```python
from build123d import *

# Parameters (mm, degrees)
F0_W     = 25.4
F0_H     = 30.48
F1_DEPTH = 317.5
F0_W_2   = 20.8801385015
F0_H_2   = 34.5365251615
F2_DEPTH = 254
F3_R     = 76.2


with BuildPart() as f1:
    # F0 (on Front) → F1 (new body)
    with BuildSketch(Plane.XZ):
        Polygon((0, 121.8727435376), (-95.25, 62.9464942231), (95.25, 62.9464942231), align=None)
        Polygon((95.25, 62.9464942231), (-95.25, 62.9464942231), (-95.25, -62.9464942231), (-20.8801385015, -62.9464942231), (-20.8801385015, -28.4099690616), (0, -28.4099690616), (0, -62.9464942231), (95.25, -62.9464942231), align=None)
        with Locations((-49.3217527476, -33.6759798229)):
            Rectangle(F0_W, F0_H, mode=Mode.SUBTRACT)
        with Locations((52.5188967586, -33.6759798229)):
            Rectangle(F0_W, F0_H, mode=Mode.SUBTRACT)
        with Locations((-49.3217527476, 34.4667454919)):
            Rectangle(F0_W, F0_H, mode=Mode.SUBTRACT)
        with Locations((52.5188967586, 34.0303108096)):
            Rectangle(F0_W, F0_H, mode=Mode.SUBTRACT)
    extrude(amount=F1_DEPTH)

    # F0 (on Front) → F2 (join)
    with BuildSketch(Plane.XZ):
        with Locations((52.5188967586, 34.0303108096)):
            Rectangle(F0_W, F0_H)
        with Locations((-49.3217527476, 34.4667454919)):
            Rectangle(F0_W, F0_H)
        with Locations((52.5188967586, -33.6759798229)):
            Rectangle(F0_W, F0_H)
        with Locations((-49.3217527476, -33.6759798229)):
            Rectangle(F0_W, F0_H)
        with Locations((-10.4400692508, -45.6782316424)):
            Rectangle(F0_W_2, F0_H_2)
    extrude(amount=F2_DEPTH)

    # F3
    f3_edges = [f1.edges().sort_by_distance(p)[0] for p in [
        (0, -158.75, 121.872744),
    ]]
    fillet(f3_edges, radius=F3_R)


solid = f1.part
```
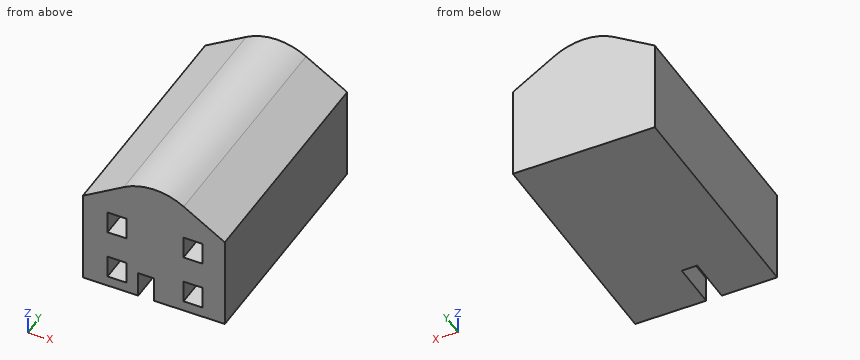
Part model, mm, in its own coordinate system. Give positions to 0.01 mm unless a question says otherwise; leave off trailing zeros. Order: outer loops, then holes, each group sorted by start corner. A loop starts at its lowest first (then second) coordinate and runs counter-clockwise, first axis right, second up. Notation, with made-up numbers: M 22.5,-16 L 39.5,-16 A38 cw 39.5,22 Z; hole C 50,-36 d6. An arc over 180 degrees is marked long. Use a Markdown table: item, result. Add a question column.
(1) Saw through at C-C, the plane x = 51.5. Give the cut face in (y, z), and give its area (3 significant figures).
(2) Drop flat-ended pins along their axis: P1, Ø3, axis at x = -20.5, y = -259.5, coming from the +Z side; P2, Ø2, axis at x = -74, y = -194, coming from the +Z side; P3, Ø12.5, axis at x = -53, y = -289, coming from the +Z side; P4, Ø4, axis at x = 58, z = 90, coming from the -Y side. Give the stop position or say it passes through.
(3) Saw through at B-B, the plane z = -25. Give the cut face in (x, y), and give its area (3 significant figures).
(4) Saw through at D-D, the plane z = 74.5. Give the cut face in (x, y), and give its area (3 significant figures).
(5) Probe line 1 along Y through (x, z) = (-14, -49); line 2 along Z through (x, y) = (12, -236.5); line 3 along Z through (x, y) = (-11.5, -59.5). List the from-to ranges inside material, lowest first. Write a range as [from, to].
(6) Saw through at A-A, the plane y = -94. Give the cut face in (x, z).
Answer key:
| question | item | result |
|---|---|---|
| 1 | outline | M -317.5,-62.95 L 0,-62.95 L 0,90.01 L -317.5,90.01 L -317.5,49.27 L -254,49.27 L -254,18.79 L -317.5,18.79 L -317.5,-18.44 L -254,-18.44 L -254,-48.92 L -317.5,-48.92 Z |
| 1 | area | 44,700 mm^2 |
| 2 | P1 | z = 106.06 |
| 2 | P2 | z = 76.71 |
| 2 | P3 | z = 92.95 |
| 2 | P4 | through |
| 3 | outline | M -95.25,-317.5 L -62.02,-317.5 L -62.02,-254 L -36.62,-254 L -36.62,-317.5 L 39.82,-317.5 L 39.82,-254 L 65.22,-254 L 65.22,-317.5 L 95.25,-317.5 L 95.25,0 L -95.25,0 Z |
| 3 | area | 57,300 mm^2 |
| 4 | outline | M -76.57,-317.5 L 76.57,-317.5 L 76.57,0 L -76.57,0 Z |
| 4 | area | 48,600 mm^2 |
| 5 | line 1 | [-254, 0] |
| 5 | line 2 | [-62.95, 107.52] |
| 5 | line 3 | [-62.95, 107.6] |
| 6 | outline | M -95.25,-62.95 L 95.25,-62.95 L 95.25,62.95 L 40.09,97.07 A76.2 ccw -40.09,97.07 L -95.25,62.95 Z |
